Geometry: final body of the model. Coordinates: model frame, mm. Face numbers are marked on the shaded views. Round coordinates to 2 decimals unless told otherwise and drop trailing zeros. Write each loop counter-clockwise with the first axis right and the second up, starting at its lowest first coordinate (ties: lowest second). Pieces come first, ordered by that corner, then holes. Notation, with made-up numbers: (16, 20) -> (52, 20) arc R23 ccw to (52, 56) -> close; hole circle Ø3 at (-11.75, 84). An arc over 180 degrees is marked (long way). Use one line per item in the form item = value. Start each with the question number.
1. Line query: L1, parallel to Y at x = -30, z = -103; L2, parallel to X at y = -133, z = -48; L3, parallel to X at y = 10, z = -108. Output: solid intervals per line, ascending.
2. Cut plane A-A, the plane z = -49. Return the cut outline in (x, y), plus the area to 3 significant figures.
3. Draft query along X for the marked faces 1, 2 and 3. Return one class per face: pulls with the +X half, pulls with the -X half, needs draft (parallel to the pull), parting line crosses it, or undercut.
4. Cut plane C-C, the plane x = 160. Return the cut outline in (y, z).
5. Cut plane B-B, the plane y = -172. Return the cut outline in (x, z).
6. Cut plane D-D, the plane z = -152. Return the cut outline in (x, y).
7. Pin query (flat end, axial travel): pin 1 Ø11 at (y, z) = (-128, -63.5) entering from +X; pin 2 Ø4 at (x, z) = (-148, -49) entering from +Y; pin 3 Ø2 at (y, z) = (-193.5, 3) entering from +X. Return the tip coordinate at first contact, or that it passes through.
```python
from build123d import *

# Parameters (mm, degrees)
F0_W      = 400
F0_H      = 400
F3_T      = -10
F4_W      = 391.7157287525
F4_H      = 391.7157287525
F4_W_2    = 383.7157287525
F4_H_2    = 383.7157287525
F5_DEPTH  = 8
F10_DEPTH = 288.5005667948
F11_DEPTH = 288.5005667948
F12_DEPTH = 288.5005667948
F13_DEPTH = 288.5005667948
F14_W     = 25
F14_H     = 8
F15_DEPTH = 395.8588644763
F16_W     = 25
F16_H     = 8
F17_DEPTH = 395.8588644763


with BuildPart() as f2:
    # F0 (on Top) → F2 section 0
    with BuildSketch(Plane.XY, mode=Mode.PRIVATE) as f2_s0:
        Rectangle(F0_W, F0_H)
    loft([f2_s0.sketch, Vertex(0, 0, -200)])

    # F3
    f3_openings = [f2.faces().sort_by_distance(p)[0] for p in [
        (0, 0, 0),
    ]]
    offset(amount=F3_T, openings=f3_openings)

    # F4 (on face) → F5 (join)
    with BuildSketch(Plane.XY):
        Rectangle(F4_W, F4_H)
        Rectangle(F4_W_2, F4_H_2, mode=Mode.SUBTRACT)
    extrude(amount=F5_DEPTH)

    # F6 (on face) → F10 (cut, through all)
    with BuildSketch(Plane(origin=(0, -100, -100), x_dir=(1, 0, 0), z_dir=(0, -0.7071067812, -0.7071067812))):
        with BuildLine():
            ThreePointArc((-7.2284161474, 44.5786437627), (-4.5414755311, 40.6099755695), (0, 39.0786437627))
            Line((0, 39.0786437627), (0, 44.5786437627))
            Line((0, 44.5786437627), (-7.2284161474, 44.5786437627))
        make_face()
        with BuildLine():
            Line((0, 44.5786437627), (0, 39.0786437627))
            ThreePointArc((0, 39.0786437627), (4.5414755311, 40.6099755695), (7.2284161474, 44.5786437627))
            Line((7.2284161474, 44.5786437627), (0, 44.5786437627))
        make_face()
        with BuildLine():
            Line((-7.2284161474, 44.5786437627), (0, 44.5786437627))
            Line((0, 44.5786437627), (0, 46.5786437627))
            Line((0, 46.5786437627), (7.5, 46.5786437627))
            ThreePointArc((7.5, 46.5786437627), (7.4317938987, 47.5878213721), (7.2284161474, 48.5786437627))
            Line((7.2284161474, 48.5786437627), (-7.2284161474, 48.5786437627))
            ThreePointArc((-7.2284161474, 48.5786437627), (-7.5, 46.5786437627), (-7.2284161474, 44.5786437627))
        make_face()
        with BuildLine():
            Line((0, 46.5786437627), (0, 44.5786437627))
            Line((0, 44.5786437627), (7.2284161474, 44.5786437627))
            ThreePointArc((7.2284161474, 44.5786437627), (7.4317938987, 45.5694661533), (7.5, 46.5786437627))
            Line((7.5, 46.5786437627), (0, 46.5786437627))
        make_face()
        with BuildLine():
            Line((-15, 44.5786437627), (-7.2284161474, 44.5786437627))
            ThreePointArc((-7.2284161474, 44.5786437627), (-7.5, 46.5786437627), (-7.2284161474, 48.5786437627))
            Line((-7.2284161474, 48.5786437627), (-15, 48.5786437627))
            Line((-15, 48.5786437627), (-15, 44.5786437627))
        make_face()
        with BuildLine():
            ThreePointArc((7.5, 46.5786437627), (7.4317938987, 45.5694661533), (7.2284161474, 44.5786437627))
            Line((7.2284161474, 44.5786437627), (15, 44.5786437627))
            Line((15, 44.5786437627), (15, 48.5786437627))
            Line((15, 48.5786437627), (7.2284161474, 48.5786437627))
            ThreePointArc((7.2284161474, 48.5786437627), (7.4317938987, 47.5878213721), (7.5, 46.5786437627))
        make_face()
        with BuildLine():
            ThreePointArc((7.2284161474, 48.5786437627), (0, 54.0786437627), (-7.2284161474, 48.5786437627))
            Line((-7.2284161474, 48.5786437627), (7.2284161474, 48.5786437627))
        make_face()
    extrude(amount=-F10_DEPTH, mode=Mode.SUBTRACT)

    # F7 (on face) → F11 (cut, through all)
    with BuildSketch(Plane(origin=(100, 0, -100), x_dir=(0, 1, 0), z_dir=(0.7071067812, 0, -0.7071067812))):
        with BuildLine():
            ThreePointArc((-7.2284161474, 44.5786437627), (-4.5414755311, 40.6099755695), (0, 39.0786437627))
            Line((0, 39.0786437627), (0, 44.5786437627))
            Line((0, 44.5786437627), (-7.2284161474, 44.5786437627))
        make_face()
        with BuildLine():
            Line((0, 44.5786437627), (0, 39.0786437627))
            ThreePointArc((0, 39.0786437627), (4.5414755311, 40.6099755695), (7.2284161474, 44.5786437627))
            Line((7.2284161474, 44.5786437627), (0, 44.5786437627))
        make_face()
        with BuildLine():
            Line((-7.2284161474, 44.5786437627), (0, 44.5786437627))
            Line((0, 44.5786437627), (0, 46.5786437627))
            Line((0, 46.5786437627), (7.5, 46.5786437627))
            ThreePointArc((7.5, 46.5786437627), (7.4317938987, 47.5878213721), (7.2284161474, 48.5786437627))
            Line((7.2284161474, 48.5786437627), (-7.2284161474, 48.5786437627))
            ThreePointArc((-7.2284161474, 48.5786437627), (-7.5, 46.5786437627), (-7.2284161474, 44.5786437627))
        make_face()
        with BuildLine():
            Line((0, 46.5786437627), (0, 44.5786437627))
            Line((0, 44.5786437627), (7.2284161474, 44.5786437627))
            ThreePointArc((7.2284161474, 44.5786437627), (7.4317938987, 45.5694661533), (7.5, 46.5786437627))
            Line((7.5, 46.5786437627), (0, 46.5786437627))
        make_face()
        with BuildLine():
            Line((-15, 44.5786437627), (-7.2284161474, 44.5786437627))
            ThreePointArc((-7.2284161474, 44.5786437627), (-7.5, 46.5786437627), (-7.2284161474, 48.5786437627))
            Line((-7.2284161474, 48.5786437627), (-15, 48.5786437627))
            Line((-15, 48.5786437627), (-15, 44.5786437627))
        make_face()
        with BuildLine():
            ThreePointArc((7.5, 46.5786437627), (7.4317938987, 45.5694661533), (7.2284161474, 44.5786437627))
            Line((7.2284161474, 44.5786437627), (15, 44.5786437627))
            Line((15, 44.5786437627), (15, 48.5786437627))
            Line((15, 48.5786437627), (7.2284161474, 48.5786437627))
            ThreePointArc((7.2284161474, 48.5786437627), (7.4317938987, 47.5878213721), (7.5, 46.5786437627))
        make_face()
        with BuildLine():
            ThreePointArc((7.2284161474, 48.5786437627), (0, 54.0786437627), (-7.2284161474, 48.5786437627))
            Line((-7.2284161474, 48.5786437627), (7.2284161474, 48.5786437627))
        make_face()
    extrude(amount=-F11_DEPTH, mode=Mode.SUBTRACT)

    # F8 (on face) → F12 (cut, through all)
    with BuildSketch(Plane(origin=(0, 100, -100), x_dir=(-1, 0, 0), z_dir=(0, 0.7071067812, -0.7071067812))):
        with BuildLine():
            ThreePointArc((-7.2284161474, 44.5786437627), (-4.5414755311, 40.6099755695), (0, 39.0786437627))
            Line((0, 39.0786437627), (0, 44.5786437627))
            Line((0, 44.5786437627), (-7.2284161474, 44.5786437627))
        make_face()
        with BuildLine():
            Line((0, 44.5786437627), (0, 39.0786437627))
            ThreePointArc((0, 39.0786437627), (4.5414755311, 40.6099755695), (7.2284161474, 44.5786437627))
            Line((7.2284161474, 44.5786437627), (0, 44.5786437627))
        make_face()
        with BuildLine():
            Line((-7.2284161474, 44.5786437627), (0, 44.5786437627))
            Line((0, 44.5786437627), (0, 46.5786437627))
            Line((0, 46.5786437627), (7.5, 46.5786437627))
            ThreePointArc((7.5, 46.5786437627), (7.4317938987, 47.5878213721), (7.2284161474, 48.5786437627))
            Line((7.2284161474, 48.5786437627), (-7.2284161474, 48.5786437627))
            ThreePointArc((-7.2284161474, 48.5786437627), (-7.5, 46.5786437627), (-7.2284161474, 44.5786437627))
        make_face()
        with BuildLine():
            Line((0, 46.5786437627), (0, 44.5786437627))
            Line((0, 44.5786437627), (7.2284161474, 44.5786437627))
            ThreePointArc((7.2284161474, 44.5786437627), (7.4317938987, 45.5694661533), (7.5, 46.5786437627))
            Line((7.5, 46.5786437627), (0, 46.5786437627))
        make_face()
        with BuildLine():
            Line((-15, 44.5786437627), (-7.2284161474, 44.5786437627))
            ThreePointArc((-7.2284161474, 44.5786437627), (-7.5, 46.5786437627), (-7.2284161474, 48.5786437627))
            Line((-7.2284161474, 48.5786437627), (-15, 48.5786437627))
            Line((-15, 48.5786437627), (-15, 44.5786437627))
        make_face()
        with BuildLine():
            ThreePointArc((7.5, 46.5786437627), (7.4317938987, 45.5694661533), (7.2284161474, 44.5786437627))
            Line((7.2284161474, 44.5786437627), (15, 44.5786437627))
            Line((15, 44.5786437627), (15, 48.5786437627))
            Line((15, 48.5786437627), (7.2284161474, 48.5786437627))
            ThreePointArc((7.2284161474, 48.5786437627), (7.4317938987, 47.5878213721), (7.5, 46.5786437627))
        make_face()
        with BuildLine():
            ThreePointArc((7.2284161474, 48.5786437627), (0, 54.0786437627), (-7.2284161474, 48.5786437627))
            Line((-7.2284161474, 48.5786437627), (7.2284161474, 48.5786437627))
        make_face()
    extrude(amount=-F12_DEPTH, mode=Mode.SUBTRACT)

    # F9 (on face) → F13 (cut, through all)
    with BuildSketch(Plane(origin=(-100, 0, -100), x_dir=(0.7071067812, 0, -0.7071067812), z_dir=(-0.7071067812, 0, -0.7071067812))):
        with BuildLine():
            ThreePointArc((-44.5786437627, -7.2284161474), (-40.6099755695, -4.5414755311), (-39.0786437627, 0))
            Line((-39.0786437627, 0), (-44.5786437627, 0))
            Line((-44.5786437627, 0), (-44.5786437627, -7.2284161474))
        make_face()
        with BuildLine():
            Line((-44.5786437627, 0), (-39.0786437627, 0))
            ThreePointArc((-39.0786437627, 0), (-40.6099755695, 4.5414755311), (-44.5786437627, 7.2284161474))
            Line((-44.5786437627, 7.2284161474), (-44.5786437627, 0))
        make_face()
        with BuildLine():
            Line((-44.5786437627, -7.2284161474), (-44.5786437627, 0))
            Line((-44.5786437627, 0), (-44.5786437627, 7.2284161474))
            ThreePointArc((-44.5786437627, 7.2284161474), (-46.5786437627, 7.5), (-48.5786437627, 7.2284161474))
            Line((-48.5786437627, 7.2284161474), (-48.5786437627, -7.2284161474))
            ThreePointArc((-48.5786437627, -7.2284161474), (-46.5786437627, -7.5), (-44.5786437627, -7.2284161474))
        make_face()
        with BuildLine():
            ThreePointArc((-48.5786437627, 7.2284161474), (-46.5786437627, 7.5), (-44.5786437627, 7.2284161474))
            Line((-44.5786437627, 7.2284161474), (-44.5786437627, 15))
            Line((-44.5786437627, 15), (-48.5786437627, 15))
            Line((-48.5786437627, 15), (-48.5786437627, 7.2284161474))
        make_face()
        with BuildLine():
            Line((-44.5786437627, -15), (-44.5786437627, -7.2284161474))
            ThreePointArc((-44.5786437627, -7.2284161474), (-46.5786437627, -7.5), (-48.5786437627, -7.2284161474))
            Line((-48.5786437627, -7.2284161474), (-48.5786437627, -15))
            Line((-48.5786437627, -15), (-44.5786437627, -15))
        make_face()
        with BuildLine():
            Line((-48.5786437627, -7.2284161474), (-48.5786437627, 7.2284161474))
            ThreePointArc((-48.5786437627, 7.2284161474), (-54.0786437627, 0), (-48.5786437627, -7.2284161474))
        make_face()
    extrude(amount=-F13_DEPTH, mode=Mode.SUBTRACT)

    # F14 (on face) → F15 (cut, through all)
    with BuildSketch(Plane.XZ.offset(195.8578643763)):
        with Locations((-12.5, 4)):
            Rectangle(F14_W, F14_H)
        with Locations((12.5, 4)):
            Rectangle(F14_W, F14_H)
    extrude(amount=-F15_DEPTH, mode=Mode.SUBTRACT)

    # F16 (on face) → F17 (cut, through all)
    with BuildSketch(Plane(origin=(-195.8578643763, 0, 0), x_dir=(0, -1, 0), z_dir=(-1, 0, 0))):
        with Locations((-12.5, 4)):
            Rectangle(F16_W, F16_H)
        with Locations((12.5, 4)):
            Rectangle(F16_W, F16_H)
    extrude(amount=-F17_DEPTH, mode=Mode.SUBTRACT)


solid = f2.part
```
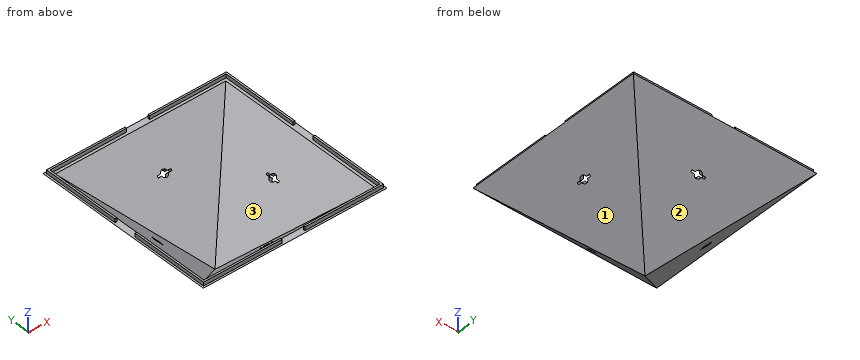
Outcome:
q1.L1 = -97 to -82.86, 82.86 to 97
q1.L2 = -152 to -137.86, 137.86 to 152
q1.L3 = -92 to -77.86, 77.86 to 92
q2.outline = (-151, -151) -> (151, -151) -> (151, 151) -> (-151, 151) -> close; hole (-136.86, -136.86) -> (136.86, -136.86) -> (136.86, 136.86) -> (-136.86, 136.86) -> close
q2.area = 16,300 mm^2
q3.face_1 = pulls with the +X half
q3.face_2 = needs draft
q3.face_3 = undercut
q4.outline = (-200, 0) -> (-160, -40) -> (160, -40) -> (200, 0) -> (195.86, 0) -> (195.86, 8) -> (191.86, 8) -> (191.86, 0) -> (185.86, 0) -> (160, -25.86) -> (-160, -25.86) -> (-185.86, 0) -> (-191.86, 0) -> (-191.86, 8) -> (-195.86, 8) -> (-195.86, 0) -> close
q5.outline = (-200, 0) -> (-172, -28) -> (172, -28) -> (200, 0) -> (195.86, 0) -> (195.86, 8) -> (191.86, 8) -> (191.86, 0) -> (185.86, 0) -> (172, -13.86) -> (-172, -13.86) -> (-185.86, 0) -> (-191.86, 0) -> (-191.86, 8) -> (-195.86, 8) -> (-195.86, 0) -> close
q6.outline = (-48, -48) -> (48, -48) -> (48, 48) -> (-48, 48) -> close; hole (-33.86, -33.86) -> (33.86, -33.86) -> (33.86, 33.86) -> (-33.86, 33.86) -> close
q7.pin_1 = 142
q7.pin_2 = 153
q7.pin_3 = 195.86
